Autodesk Inventor part; units mm, degrees
ref_plane "Work Plane1" through (0, 6.35, 0) normal (0, 1, 0) x (1, 0, 0)
ref_plane "YZ Plane" through (0, 0, 0) normal (1, 0, 0) x (0, 1, 0)
ref_plane "XZ Plane" through (0, 0, 0) normal (0, 1, 0) x (-1, 0, 0)
sketch "Sketch1" plane through (0, 0, 0) normal (0, 1, 0) x (-1, 0, 0)
  circle A0 centre (254, -50.8) radius 14.2875
  arc A1 (38.4735, -38.1055) -> (38.4735, -63.4945) centre (38.1, -50.8) ccw
  line L0 (280.9875, -50.8) -> (280.9875, 0)
  line L1 (280.9875, 0) -> (280.9875, -50.8)
  line L2 (280.9875, 0) -> (38.1, 0)
  line L3 (38.1, -38.1) -> (38.1, 0)
  arc A2 (38.4735, -63.4945) -> (43.8871, -100.4525) centre (254, -50.8) ccw
  arc A3 (51.1687, -124.7749) -> (66.9545, -158.6276) centre (254, -50.8) ccw
  arc A4 (80.906, -179.8398) -> (105.7377, -207.743) centre (254, -50.8) ccw
  arc A5 (273.4803, -69.4773) -> (280.9875, -50.8) centre (254, -50.8) ccw
  line L4 (125.2338, -224.0976) -> (273.4803, -69.4773)
  line L5 (280.9875, 0) -> (38.1, 0)
  line L6 (38.1, 0) -> (38.1, -38.1)
  line L7 (280.9875, 0) -> (280.9875, -50.8)
  circle A6 centre (47.1701, -112.7208) radius 6.35
  circle A7 centre (38.1, -50.8) radius 6.35
  arc A8 (43.8871, -100.4525) -> (51.1687, -124.7749) centre (47.1701, -112.7208) ccw
  arc A9 (38.4735, -38.1055) -> (38.4735, -63.4945) centre (38.1, -50.8) ccw
  arc A10 (43.8871, -100.4525) -> (51.1687, -124.7749) centre (47.1701, -112.7208) ccw
  line L8 (38.1, 0) -> (50.8, 0)
  line L9 (38.4739, -38.1) -> (38.1, -38.1)
  line L10 (38.1, -38.1) -> (38.1, 0)
  circle A11 centre (254, -50.8) radius 14.2875
  circle A12 centre (47.1701, -112.7208) radius 6.35
  circle A13 centre (38.1, -50.8) radius 6.35
  arc A14 (51.1687, -124.7749) -> (125.2338, -224.0976) centre (254, -50.8) ccw
  arc A15 (38.1934, -57.1493) -> (43.8871, -100.4525) centre (254, -50.8) ccw
  arc A16 (35.0036, -116.3632) -> (116.3789, -233.3332) centre (254, -50.8) ccw
  line L11 (125.2338, -224.0976) -> (116.3789, -233.3332)
  point P0 (0, 0)
  point P1 (44.1616, 0)
  point P2 (38.1934, -44.4507)
  dimension "d4" = 28.575
  dimension "d32" = 25.4
  dimension "d36" = 50.8
  dimension "d74" = 53.975
  dimension "d79" = 12.7
  dimension "d83" = 26.9875
ref_plane "Work Plane1" through (0, 6.35, 0) normal (0, 1, 0) x (1, 0, 0)
extrude "Extrusion7" add sketch "Sketch1" along normal blind 6.35
sketch "Sketch4" plane through (0, 6.35, 0) normal (0, 1, 0) x (1, 0, 0)
  arc A0 (-116.4883, 215.1788) -> (-120.5628, 210.3083) centre (-118.5256, 212.7436) ccw
  arc A1 (-116.4883, 215.1788) -> (-120.5628, 210.3083) centre (-118.5256, 212.7436) ccw
  arc A2 (-60.849, 127.8786) -> (-54.9513, 130.2322) centre (-57.9002, 129.0554) ccw
  arc A3 (-60.849, 127.8786) -> (-54.9513, 130.2322) centre (-57.9002, 129.0554) ccw
  circle A4 centre (-254, 50.8) radius 14.2875
  arc A5 (-54.9513, 130.2322) -> (-116.4883, 215.1788) centre (-254, 50.8) ccw
  arc A6 (-54.9513, 130.2322) -> (-116.4883, 215.1788) centre (-254, 50.8) ccw
  arc A7 (-60.849, 127.8786) -> (-120.5628, 210.3083) centre (-254, 50.8) ccw
  point P0 (0, 0)
extrude "Extrusion9" cut sketch "Sketch4" against normal blind 3.175 contours A5 A2 A7 A0
sketch "Sketch5" plane through (0, 3.175, 0) normal (0, 1, 0) x (1, 0, 0)
  arc A0 (-116.4883, 215.1788) -> (-120.5628, 210.3083) centre (-118.5256, 212.7436) ccw
  circle A1 centre (-118.5256, 212.7436) radius 3.175
  point P0 (0, 0)
extrude "Extrusion10" add sketch "Sketch5" along normal blind 19.05
sketch "Sketch6" plane through (-118.5256, 22.225, -212.7436) normal (0, 1, 0) x (1, 0, 0)
  arc A0 (2.0372, 2.4352) -> (-2.0372, -2.4352) centre (0, 0) ccw
  circle A1 centre (0, 0) radius 6.35
  point P0 (118.5256, -212.7436)
  dimension "d110" = 12.7
extrude "Extrusion11" add sketch "Sketch6" against normal blind 6.35
properties part number "Hood panel" material "Aluminum 6061"
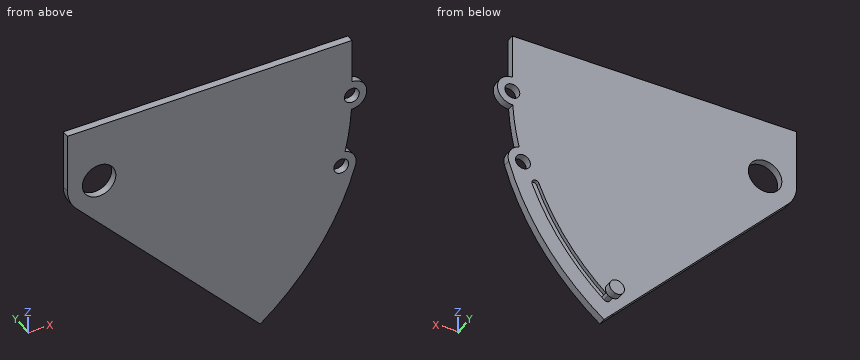
For this review, take the finished solid that the model builds, in its own axes (mm). Round coordinates to 2 decimals unless told otherwise and drop trailing zeros. Order: outer loops, then holes, each group sorted by start corner. A loop starts at its lowest first (then second) coordinate and runs counter-clockwise, first axis right, second up.
Q1. Insertion check: P1, Ø3, axis at y = 2.5, z = -18, coming from the +X side; P2, Ø6, axis at x = -171.5, z = -53, coming from the +Y side. Each pin has a flat end and moves straight along its axis. Give the tip position at first contact, or say it passes through.
Findings below:
P1: stops at x = -38.1
P2: stops at y = 6.35
Q2. We need section D-D, the plane y = 12.5. Give the boundary of the cut face in (x, z) (3 decimals), plus the area to 3 significant figures.
Findings below:
outline: (-120.563, -210.308) arc R3.175 ccw to (-116.488, -215.179) arc R3.175 ccw to start
area: 31.7 mm2
Q3. We need section C-C, the plane z = -122.5. Give the boundary of the cut face in (x, y).
Findings below:
outline: (-222.64, 0) - (-36.94, 0) - (-36.94, 6.35) - (-222.64, 6.35) - close
Q4. Wall thickness on line 1 (Y direction, x = -50, z = -93.5); line 2 (Z direction, x = -246.5, y = 2); line 3 (Z direction, x = -254, y = 1.75): over which ranges is each line inside the solid? List them lowest first.
Findings below:
line 1: y = 0 to 6.35
line 2: z = -97.62 to -62.96, -38.64 to 0
line 3: z = -89.8 to -65.09, -36.51 to 0
Q5. We need section A-A, the plane x = -254. Give the boundary of the cut face in (y, z), plus the area to 3 significant figures.
Findings below:
outline: (0, -89.8) - (6.35, -89.8) - (6.35, -65.09) - (0, -65.09) - close; (0, -36.51) - (6.35, -36.51) - (6.35, 0) - (0, 0) - close
area: 389 mm2
Q6. We need section B-B, the plane x = -67.5. Give the boundary of the cut face in (y, z) (3 decimals), plus the area to 3 significant figures.
Findings below:
outline: (0, -182.996) - (6.35, -182.996) - (6.35, -156.382) - (3.175, -156.382) - (3.175, -142.812) - (6.35, -142.812) - (6.35, 0) - (0, 0) - close
area: 1,120 mm2
